from build123d import *

# Parameters (mm, degrees)
BOSS_EXTRUDE1_DEPTH = 10
SKETCH2_3_W         = 10
SKETCH2_3_H         = 20
BOSS_EXTRUDE2_DEPTH = 20
BOSS_EXTRUDE3_START = -10
BOSS_EXTRUDE3_DEPTH = 10
SKETCH8_R           = 3
BOSS_EXTRUDE5_DEPTH = 0.1
DOME2_FACE_RADIUS   = 3
DOME2_HEIGHT        = 4
DOME3_FACE_RADIUS   = 3
DOME3_HEIGHT        = 4
FILLET1_RADIUS      = 5
FILLET1_LENGTH      = 20
FILLET2_RADIUS      = 5
FILLET2_LENGTH      = 20
FILLET3_R           = 10
FILLET4_R           = 10


# Read off the part's stored shape, not the designer's step: Boss-Extrude3
with BuildPart() as part:
    # Sketch2 → Boss-Extrude1 (new body)
    with BuildSketch(Plane(origin=(0, 0, 0), x_dir=(1, 0, 0), z_dir=(0, 1, 0))):
        Polygon((-10, 45), (-50, 45), (-50, -45), (-10, -45), (-10, -25), (-10, 25), align=None)
    extrude(amount=BOSS_EXTRUDE1_DEPTH)

    # Sketch2<3> → Boss-Extrude2 (add)
    with BuildSketch(Plane(origin=(0, 0, 0), x_dir=(1, 0, 0), z_dir=(0, 1, 0))):
        with Locations((-5, -35)):
            Rectangle(SKETCH2_3_W, SKETCH2_3_H)
        with Locations((-5, 35)):
            Rectangle(SKETCH2_3_W, SKETCH2_3_H)
    extrude(amount=BOSS_EXTRUDE2_DEPTH)

    # Boss-Extrude3 outline → Boss-Extrude3 (add)
    with BuildSketch(Plane(origin=(-16.160254038, -4.330127019, 0), x_dir=(0, 0, -1), z_dir=(0.9659258262890681, 0.25881904510252135, 0)).offset(BOSS_EXTRUDE3_START)):
        with BuildLine():
            Line((-45, 114.835639165), (-45, 14.835639165))
            Line((-45, 14.835639165), (-39, 14.835639165))
            Line((-39, 14.835639165), (-39, 59.835639165))
            Line((-39, 59.835639165), (-39, 69.835639165))
            Line((-39, 69.835639165), (-39, 114.835639165))
            ThreePointArc((-39, 114.835639165), (-42, 117.835639165), (-45, 114.835639165))
        make_face()
        with BuildLine():
            Line((-39, 69.835639165), (-39, 59.835639165))
            add(Edge.make_bspline(
                [(-39, 59.835639165), (-32.29466778, 59.812740608), (-23.746310881, 57.26615983), (-18.155959882, 54.002687415), (-13.581360263, 49.447869434), (-9.895970778, 43.393937355), (-7.1466079, 35.668544709), (-5.009950643, 23.851055873), (-5, 14.835639165)],
                knots=[0, 0, 0, 0.1875, 0.3125, 0.4375, 0.5625, 0.6875, 0.8125, 1, 1, 1], degree=2))
            Line((-5, 14.835639165), (5, 14.835639165))
            add(Edge.make_bspline(
                [(0.000646167, 45.244430902), (0.476875904, 44.083141287), (2.5762954, 38.143358621), (5.009950643, 24.570222457), (5, 14.835639165)],
                knots=[0.655563959, 0.655563959, 0.655563959, 0.6875, 0.8125, 1, 1, 1], degree=2))
            add(Edge.make_bspline(
                [(0.000646167, 45.244430902), (0.000323073, 45.243642557), (0, 45.24285419)],
                knots=[0.655550731, 0.655550731, 0.655550731, 0.655572405, 0.655572405, 0.655572405], degree=2))
            add(Edge.make_bspline(
                [(-39, 69.835639165), (-31.080450951, 69.858370058), (-19.824359781, 66.54538789), (-12.00867454, 61.996263654), (-5.614755257, 55.613542625), (-1.387837079, 48.627543749), (0, 45.24285419)],
                knots=[0, 0, 0, 0.1875, 0.3125, 0.4375, 0.5625, 0.655579399, 0.655579399, 0.655579399], degree=2))
        make_face()
        with BuildLine():
            add(Edge.make_bspline(
                [(39, 69.835639165), (36.362179487, 69.835639165), (28.828562218, 69.197832663), (19.824098622, 66.545415855), (12.008024479, 61.996828001), (5.61432407, 55.613689023), (1.991176128, 49.630689625), (0.466161192, 46.380278102), (0.000646167, 45.244430902)],
                knots=[0, 0, 0, 0.0625, 0.1875, 0.3125, 0.4375, 0.5625, 0.624322405, 0.655550731, 0.655550731, 0.655550731], degree=2))
            add(Edge.make_bspline(
                [(0.000646167, 45.244430902), (0.476875904, 44.083141287), (2.5762954, 38.143358621), (5.009950643, 24.570222457), (5, 14.835639165)],
                knots=[0.655563959, 0.655563959, 0.655563959, 0.6875, 0.8125, 1, 1, 1], degree=2))
            add(Edge.make_bspline(
                [(39, 59.835639165), (32.29466778, 59.812740608), (23.746310881, 57.26615983), (18.155959882, 54.002687415), (13.581360263, 49.447869434), (9.895970778, 43.393937355), (7.1466079, 35.668544709), (5.009950643, 23.851055873), (5, 14.835639165)],
                knots=[0, 0, 0, 0.1875, 0.3125, 0.4375, 0.5625, 0.6875, 0.8125, 1, 1, 1], degree=2))
            Line((39, 59.835639165), (39, 69.835639165))
        make_face()
        with BuildLine():
            Line((39, 114.835639165), (39, 69.835639165))
            Line((39, 69.835639165), (39, 59.835639165))
            Line((39, 59.835639165), (39, 14.835639165))
            Line((39, 14.835639165), (45, 14.835639165))
            Line((45, 14.835639165), (43.851535226, 117.196108886))
            ThreePointArc((43.851535226, 117.196108886), (40.687484415, 117.533286814), (39, 114.835639165))
        make_face()
    extrude(amount=BOSS_EXTRUDE3_DEPTH)

    # Sketch8 → Boss-Extrude5 (add)
    with BuildSketch(Plane(origin=(-16.160254038, -4.330127019, 0), x_dir=(0, 0, -1), z_dir=(0.9659258262890682, 0.2588190451025214, 0))):
        with Locations(Location((-42, 114.835639165, 0), (0, 0, 90))):
            Circle(SKETCH8_R)
        with Locations(Location((42, 114.835639165, 0), (0, 0, 51.889621563))):
            Circle(SKETCH8_R)
    extrude(amount=BOSS_EXTRUDE5_DEPTH)

    # Dome2: a dome of height H over a round flat face of radius A is a cap of a sphere of radius (A * A + H * H) / (2 * H)
    dome2_r = (DOME2_FACE_RADIUS * DOME2_FACE_RADIUS + DOME2_HEIGHT * DOME2_HEIGHT) / (2 * DOME2_HEIGHT)
    dome2_base = Plane((-45.785311928, 106.618464533, 42), z_dir=(0.965925826289, 0.258819045103, 0))
    with Locations(dome2_base.offset(DOME2_HEIGHT - dome2_r)):
        dome2_ball = Sphere(dome2_r, mode=Mode.PRIVATE)
    add(split(dome2_ball, bisect_by=dome2_base, keep=Keep.TOP, mode=Mode.PRIVATE))

    # Dome3: a dome of height H over a round flat face of radius A is a cap of a sphere of radius (A * A + H * H) / (2 * H)
    dome3_r = (DOME3_FACE_RADIUS * DOME3_FACE_RADIUS + DOME3_HEIGHT * DOME3_HEIGHT) / (2 * DOME3_HEIGHT)
    dome3_base = Plane((-45.785311928, 106.618464533, -42), z_dir=(0.965925826289, 0.258819045103, 0))
    with Locations(dome3_base.offset(DOME3_HEIGHT - dome3_r)):
        dome3_ball = Sphere(dome3_r, mode=Mode.PRIVATE)
    add(split(dome3_ball, bisect_by=dome3_base, keep=Keep.TOP, mode=Mode.PRIVATE))

    # Fillet1: full round fillet: the end face becomes a half cylinder, R = half its width
    fillet1_face = Plane((-5, 20, -35), x_dir=(0, 0, -1), z_dir=(0, 1, 0))  # on the end face: x along it, z out of the body
    fillet1_slab = fillet1_face.offset(-FILLET1_RADIUS / 2) * Box(FILLET1_LENGTH, 2 * FILLET1_RADIUS, FILLET1_RADIUS, mode=Mode.PRIVATE)  # the body's end, R deep
    fillet1_round = Plane((-5, 15, -35), x_dir=(0, 1, 0), z_dir=(0, 0, -1)) * Cylinder(FILLET1_RADIUS, FILLET1_LENGTH, mode=Mode.PRIVATE)  # its axis R under the face
    add(fillet1_slab - fillet1_round, mode=Mode.SUBTRACT)

    # Fillet2: full round fillet: the end face becomes a half cylinder, R = half its width
    fillet2_face = Plane((-5, 20, 35), x_dir=(0, 0, 1), z_dir=(0, 1, 0))  # on the end face: x along it, z out of the body
    fillet2_slab = fillet2_face.offset(-FILLET2_RADIUS / 2) * Box(FILLET2_LENGTH, 2 * FILLET2_RADIUS, FILLET2_RADIUS, mode=Mode.PRIVATE)  # the body's end, R deep
    fillet2_round = Plane((-5, 15, 35), x_dir=(0, 1, 0), z_dir=(0, 0, 1)) * Cylinder(FILLET2_RADIUS, FILLET2_LENGTH, mode=Mode.PRIVATE)  # its axis R under the face
    add(fillet2_slab - fillet2_round, mode=Mode.SUBTRACT)

    # Fillet3
    fillet3_edges = [part.edges().sort_by_distance(p)[0] for p in [
        (0, 0, 35),
    ]]
    fillet(fillet3_edges, radius=FILLET3_R)

    # Fillet4
    fillet4_edges = [part.edges().sort_by_distance(p)[0] for p in [
        (0, 0, -35),
    ]]
    fillet(fillet4_edges, radius=FILLET4_R)


solid = part.part
Work out the finished part from the listing and answer in its coordinate system (mm). A direction names the side the tool comes from. Coordinates: 2 decimals unless noted, no trailing zeros. Order: outer loops, then holes, each group sorted by start corner. A loop starts at its lowest first (then second) coordinate and runs counter-clockwise, first axis right, second up. Notation, with made-up numbers: (-17, 20) - (8, 20) arc R20 cw to (8, 57) - close; hole circle Ø7 at (11, 59.25). An arc over 180 degrees is marked (long way). Put each result on its own line as item: value. Start each with the question number.
1) For a pull along Z with two mould halves and no side action, classify faces 1 (the flat face through (-10, 12, -35)), 2 (the flat face through (-5, 10, 25)), 3 (the flat face through (-25, 8, -45)) as released by +Z, released by -Z, zero draft, split by the parting line, or undercut.
2) Find section A-A (y = 86). Give the vertices of the cut face in (x, z), plus the area to 3 significant figures.
3) Find the intervals of material crossed by line 1 (Y direction, x = -48.5, z = 16.5); line 2 (Z direction, x = -31.5, y = 15.5); line 3 (X direction, y = 8.5, z = -3), in increasing order. Write a range as from..to.
4) For faces 4 (the flat face through (-5, 10, -25)), 5 (the flat face through (-38.587, 40.732, -3.107)), 6 (the flat face through (0, 12, -35)), determine the directions among +Z, -Z, +X, -X, +Y, -Y from which every point of the face is accessible in a straight line to the end or side of a thin tool.
5) Find section B-B (y = 33). State how many separate pieces and enclosed holes the cut face has, plus the area to 3 significant figures.
6) Flat-ended cylindrical pins translate along their axes: pin 1 (23.5 mm diameter, centred on x = -42.5, y = 79.5, fed in from -Z); pin 2 (22 mm diameter, centred on x = -16.5, y = 13.5, fed in from -Z); pin 3 (1.5 mm diameter, centred on y = 11.5, z = 38.5, fed in from -X). Find the tip coordinate at first contact, or state that the pin passes through.
Results list:
1. face 1: zero draft
1. face 2: undercut
1. face 3: released by -Z
2. outline: (-50.72, -44.09) - (-40.36, -44.12) - (-40.36, -39) - (-50.72, -39) - close; (-50.72, 39) - (-40.36, 39) - (-40.36, 45) - (-50.72, 45) - close
2. area: 115 mm^2
3. line 1: y = 0..10
3. line 2: z = -44.91..-39, -5.31..5.31, 39..45
3. line 3: x = -50..-10
4. face 4: +X, +Y, -Y
4. face 5: +Z, -Z, -X
4. face 6: +Z, -Z, +X, +Y, -Y
5. separate pieces: 3
5. enclosed holes: 0
5. area: 301 mm^2
6. pin 1: stops at z = -44.31
6. pin 2: stops at z = -45
6. pin 3: stops at x = -30.9
